The listing builds one solid part. Answer for the finished solid, in the listing's coordinates (mm). A direction names the side the tool comes from. Coordinates: 2 decimals unless noted, no trailing zeros. Loops run counter-clockwise (first coordinate to the right, second up) from the corner with the lowest first, then second, coordinate; pieces in that order, holes last. Notation, with made-up numbers: (-38.5, 62) - (-17.5, 62) arc R28 cw to (-17.5, 89) - close; hole circle Ø2 at (40, 11.25). An arc over 180 degrees is marked (long way). Write each question's results on one line, items separated by ' | '. Start each with the question number.
(1) Find section D-D on y = 10. State how many separate pieces and enclosed holes the cut face has, then the cut area to 3 significant figures.
(2) Determine the mould class of faces 4 (the flat face through (9.1, 5.42, -34.08)), 5 (the flat face through (-45.36, 5.42, 60.25)), 6 (the flat face through (-74.134, 5, 11)) for opening direction Z: released by +Z, released by -Z, zero draft, split by the parting line, or undercut.
(3) Find section B-B on x = 22.5. Determine the outline of the cut face in (y, z), then the cut area to 3 significant figures.
(4) Find section C-C on y = 99. Determine the outline of the cut face in (x, z), then the cut area to 3 significant figures.
(5) Given pin 1 Ø6 at (x, z) = (47.5, 5.5) entering from +Y; pin 2 Ø22 at (y, z) = (6, 0) entering from -X; pin 3 Ø8 at (x, y) = (-28.5, 22.5) entering from -Z, each flat-ended and moving along its own axis, determine where each tip first touches the part or whether it passes through.
(6) For faces 1 (the cylindrical face through (33.486, 9.86, -18.411)), 2 (the flat face through (50, 20, 10)), 3 (the cylindrical face through (57.254, 96.422, 0.412)), determine the directions among +Z, -Z, +X, -X, +Y, -Y from which every point of the face is accessible in a straight line to the end or side of a thin tool.
(7) Consider line 1 (Z direction, x = 56.55, y = 99); line 2 (X direction, y = 46, z = 19.5); line 3 (X direction, y = 20.5, z = -4). Determine where each line is inside the solid, lowest interval first. Write a range as from..to.
(8) Find section A-A on y = 48.5. Determine the outline of the cut face in (x, z).
from build123d import *

# Parameters (mm, degrees)
Y_KSEKLIK_EKSTR_ZYON1_DEPTH = 20
IZIM3_W                     = 25
IZIM3_H                     = 48.452994616
Y_KSEKLIK_EKSTR_ZYON2_DEPTH = 5
IZIM12_R                    = 3.5
KES_EKSTR_ZYON4_DEPTH       = 200
KES_EKSTR_ZYON5_DEPTH       = 200
KES_EKSTR_ZYON5_DEPTH_BACK  = 200
IZIM13_R                    = 3.5
IZIM14_R                    = 3.5
KES_EKSTR_ZYON6_DEPTH       = 150
IZIM10_W                    = 5
IZIM10_H                    = 48.452994616
Y_KSEKLIK_EKSTR_ZYON3_DEPTH = 80
IZIM15_W                    = 5
IZIM15_H                    = 48.452994616
Y_KSEKLIK_EKSTR_ZYON4_DEPTH = 5
IZIM11_R                    = 2.6
KES_EKSTR_ZYON3_DEPTH       = 5.5


with BuildPart() as part:
    # Çizim1 → Yükseklik-Ekstrüzyon1 (new body)
    with BuildSketch(Plane(origin=(0, 0, 0), x_dir=(1, 0, 0), z_dir=(0, 1, 0))):
        with BuildLine():
            Line((-74.133721197, -34.978223844), (-74.133721197, 13.474770772))
            ThreePointArc((-74.133721197, 13.474770772), (-72.124102253, 20.974770772), (-66.633721197, 26.465151829))
            Line((-66.633721197, 26.465151829), (-24.672196969, 50.691649137))
            ThreePointArc((-24.672196969, 50.691649137), (-17.172196969, 52.70126808), (-9.672196969, 50.691649137))
            Line((-9.672196969, 50.691649137), (32.289327258, 26.465151829))
            ThreePointArc((32.289327258, 26.465151829), (37.779708314, 20.974770772), (39.789327258, 13.474770772))
            Line((39.789327258, 13.474770772), (39.789327258, -34.978223844))
            ThreePointArc((39.789327258, -34.978223844), (37.779708314, -42.478223844), (32.289327258, -47.968604901))
            Line((32.289327258, -47.968604901), (-9.672196969, -72.195102209))
            ThreePointArc((-9.672196969, -72.195102209), (-17.172196969, -74.204721152), (-24.672196969, -72.195102209))
            Line((-24.672196969, -72.195102209), (-66.633721197, -47.968604901))
            ThreePointArc((-66.633721197, -47.968604901), (-72.124102253, -42.478223844), (-74.133721197, -34.978223844))
        make_face()
        with BuildLine():
            Line((-69.133721197, 13.474770772), (-69.133721197, -34.978223844))
            ThreePointArc((-69.133721197, -34.978223844), (-67.793975234, -39.978223844), (-64.133721197, -43.638477882))
            Line((-64.133721197, -43.638477882), (-22.172196969, -67.86497519))
            ThreePointArc((-22.172196969, -67.86497519), (-17.172196969, -69.204721152), (-12.172196969, -67.86497519))
            Line((-12.172196969, -67.86497519), (29.789327258, -43.638477882))
            ThreePointArc((29.789327258, -43.638477882), (33.449581295, -39.978223844), (34.789327258, -34.978223844))
            Line((34.789327258, -34.978223844), (34.789327258, 13.474770772))
            ThreePointArc((34.789327258, 13.474770772), (33.449581295, 18.474770772), (29.789327258, 22.13502481))
            Line((29.789327258, 22.13502481), (-12.172196969, 46.361522118))
            ThreePointArc((-12.172196969, 46.361522118), (-17.172196969, 47.70126808), (-22.172196969, 46.361522118))
            Line((-22.172196969, 46.361522118), (-64.133721197, 22.13502481))
            ThreePointArc((-64.133721197, 22.13502481), (-67.793975234, 18.474770772), (-69.133721197, 13.474770772))
        make_face(mode=Mode.SUBTRACT)
    extrude(amount=Y_KSEKLIK_EKSTR_ZYON1_DEPTH)

    # Çizim3 → Yükseklik-Ekstrüzyon2 (add)
    with BuildSketch(Plane(origin=(0, 20, 0), x_dir=(1, 0, 0), z_dir=(0, 1, 0))):
        with Locations((-81.633721197, -10.751726536)):
            Rectangle(IZIM3_W, IZIM3_H)
        with Locations((47.289327258, -10.751726536)):
            Rectangle(IZIM3_W, IZIM3_H)
    extrude(amount=Y_KSEKLIK_EKSTR_ZYON2_DEPTH)

    # Çizim12 → Kes-Ekstrüzyon4 (cut)
    with BuildSketch(Plane(origin=(39.789327258, 0, 0), x_dir=(0, 0, -1), z_dir=(1, 0, 0))):
        with Locations((-10.751726536, 10)):
            Circle(IZIM12_R)
    extrude(amount=-KES_EKSTR_ZYON4_DEPTH, mode=Mode.SUBTRACT)

    # Çizim13 → Kes-Ekstrüzyon5 (cut, two sides: drawn at the far end of the back side and taken through both)
    with BuildSketch(Plane(origin=(10.467209436, 0, -39.064157428), x_dir=(0.8660254037844397, 0, 0.4999999999999982), z_dir=(-0.4999999999999983, 0, 0.8660254037844398)).offset(-KES_EKSTR_ZYON5_DEPTH_BACK)):
        with Locations(Location((0.971513889, 10, 0), (0, 0, 180))):
            Circle(IZIM13_R)
    extrude(amount=KES_EKSTR_ZYON5_DEPTH + KES_EKSTR_ZYON5_DEPTH_BACK, mode=Mode.SUBTRACT)

    # Çizim14 → Kes-Ekstrüzyon6 (cut)
    with BuildSketch(Plane(origin=(-28.118177199, 0, -48.702111524), x_dir=(-0.8660254037844375, 0, 0.500000000000002), z_dir=(-0.500000000000002, 0, -0.8660254037844375))):
        with Locations((20.247422082, 10)):
            Circle(IZIM14_R)
    extrude(amount=-KES_EKSTR_ZYON6_DEPTH, mode=Mode.SUBTRACT)

    # Çizim10 → Yükseklik-Ekstrüzyon3 (add)
    with BuildSketch(Plane(origin=(0, 25, 0), x_dir=(1, 0, 0), z_dir=(0, 1, 0))):
        with Locations((57.289327258, -10.751726536)):
            Rectangle(IZIM10_W, IZIM10_H)
        with Locations((-91.633721197, -10.751726536)):
            Rectangle(IZIM10_W, IZIM10_H)
    extrude(amount=Y_KSEKLIK_EKSTR_ZYON3_DEPTH)

    # Çizim15 → Yükseklik-Ekstrüzyon4 (add)
    with BuildSketch(Plane(origin=(0, 105, 0), x_dir=(1, 0, 0), z_dir=(0, 1, 0))):
        with Locations((57.289327258, -10.751726536)):
            Rectangle(IZIM15_W, IZIM15_H)
    extrude(amount=Y_KSEKLIK_EKSTR_ZYON4_DEPTH)

    # Çizim11 → Kes-Ekstrüzyon3 (cut)
    with BuildSketch(Plane(origin=(54.789327258, 0, 0), x_dir=(0, 0, -1), z_dir=(1, 0, 0))):
        with Locations(Location((-20.750229228, 99, 0), (0, 0, 180))):
            Circle(IZIM11_R)
        with Locations(Location((-0.750229228, 99, 0), (0, 0, 180))):
            Circle(IZIM11_R)
    extrude(amount=KES_EKSTR_ZYON3_DEPTH, mode=Mode.SUBTRACT)


solid = part.part
Values:
1) separate pieces: 6 | enclosed holes: 0 | area: 1,640 mm²
2) face 4: undercut | face 5: released by +Z | face 6: zero draft
3) outline: (0, -32.12) - (20, -32.12) - (20, -26.34) - (0, -26.34) - close; (0, 47.85) - (20, 47.85) - (20, 53.62) - (0, 53.62) - close | area: 231 mm²
4) outline: (-94.13, -13.47) - (-89.13, -13.47) - (-89.13, 34.98) - (-94.13, 34.98) - close; (54.79, -13.47) - (59.79, -13.47) - (59.79, -1.85) - (54.79, -1.85) - close; (54.79, 3.35) - (59.79, 3.35) - (59.79, 18.15) - (54.79, 18.15) - close; (54.79, 23.35) - (59.79, 23.35) - (59.79, 34.98) - (54.79, 34.98) - close | area: 433 mm²
5) pin 1: stops at y = 25 | pin 2: stops at x = -74.13 | pin 3: stops at z = -50.28
6) face 1: +Y, -Y | face 2: +Z, -Z, +X, -Y | face 3: +X
7) line 1: z = -13.47..-1.85, 3.35..18.15, 23.35..34.98 | line 2: x = -94.13..-89.13, 54.79..59.79 | line 3: x = -94.13..-69.13, 34.79..59.79
8) outline: (-94.13, -13.47) - (-89.13, -13.47) - (-89.13, 34.98) - (-94.13, 34.98) - close; (54.79, -13.47) - (59.79, -13.47) - (59.79, 34.98) - (54.79, 34.98) - close
